Job drawing, mm, ordinate dimensions from the low corner. One solid piece. A direction names the side the tool comes from. Give positions to 0.01 mm unless a question says otherwise; leave off trailing zeros. Loops run counter-clockwise (first coordinate to the right, second up) from the corner with the lowest first, then second, coordinate; pieces in that order, holes last. Notation, with made-up numbers: (-23, 0) - (20, 0) arc R20 ccw to (20, 29) - close; hole circle Ø4 at (75, -38). An arc over 180 degrees is marked (long way). Answer as CSV lines item,"result". Start each with the question number.
Item 1: Pull direction X, two halves, no side cores. Call the marked faces 1, 2 and 3: pulls with the +X half, pulls with the -X half, needs draft (parallel to the pull), parting line crosses it, or undercut.
Item 2: Saw through at A-A on y = 7. Give the cut face in (x, z).
Item 3: Drill centre lines: L1, parallel to Y at x = 3, z = 0.5; L2, parallel to Y at x = 3, z = 3; L3, parallel to X at y = 11.75, z = 4.5. Where is each one in solid material? Low to high. Write a range as from..to.
Item 4: Tool access for the marked faces 4 and 5: list every direction of +Z, -Z, +X, -X, +Y, -Y with a clear straight run to the whole face (end or side of a thin tool).
Item 5: Pin check, flat tips, straight feed: pin 1 (0.9 mm diameter, centred on x = 4, z = 3.5, fed in from -Y); pin 2 (3 mm diameter, centred on y = 6, z = 4, fed in from -X). Stop position of each tip, or through.
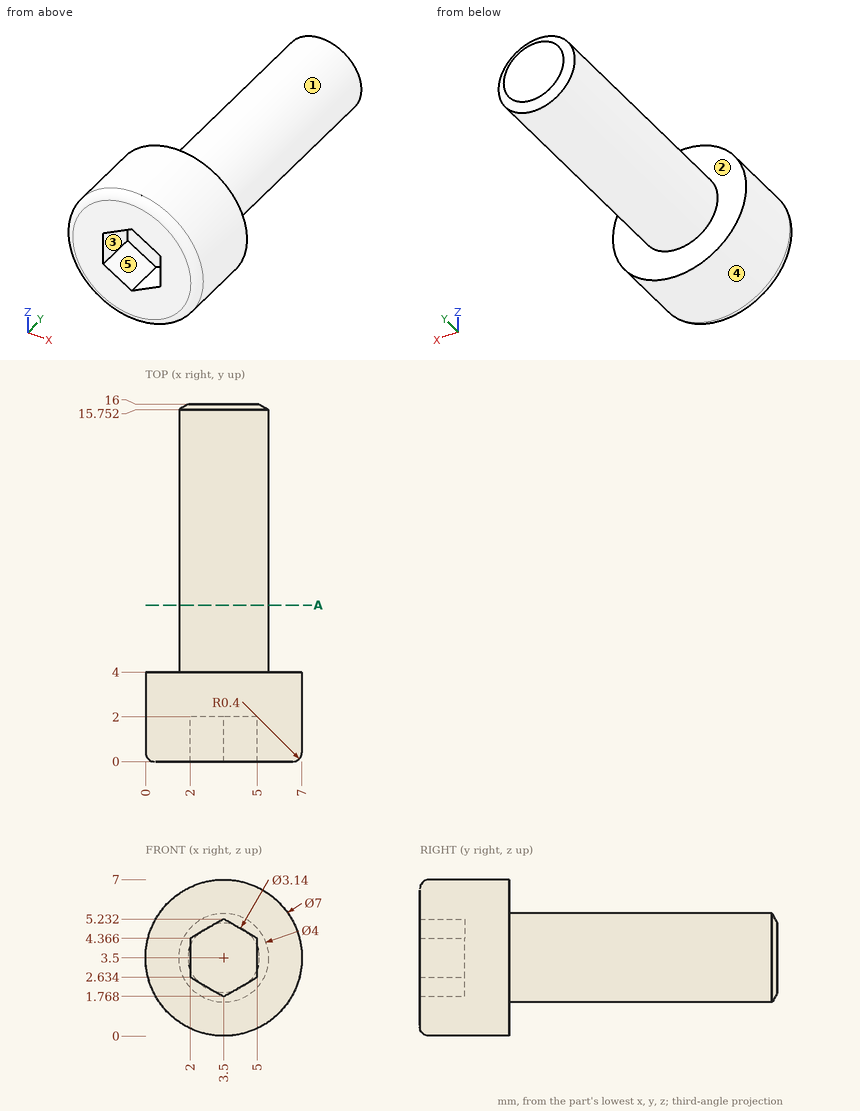
Responses:
1,face 1,"parting line crosses it"
1,face 2,"needs draft"
1,face 3,"undercut"
2,outline,"circle Ø4 at (3.5, 3.5)"
3,L1,"0..4"
3,L2,"2..16"
3,L3,"1.77..5.23"
4,face 4,"+Y, -Y"
4,face 5,"-Y"
5,pin 1,"y = 2"
5,pin 2,"x = 1.5"
